```python
from build123d import *

# Parameters (mm, degrees)
F2_R          = 1.5875
F3_DEPTH      = 19.3685
F3_DEPTH_BACK = 19.3685
F6_W          = 76.2
F6_H          = 6.35
F7_DEPTH      = 5.438244135


with BuildPart() as f1:
    # F0 (on Front) → F1 (revolve)
    with BuildSketch(Plane.XZ):
        Polygon((72.6948, 19.3675), (0, 19.3675), (0, 14.2875), (85.3948, 14.2875), (85.3948, 18.0326762121), align=None)
    revolve(axis=Axis((42.6974, 0, 0), (1, 0, 0)))

    # F2 (on Front) → F3 (cut, two sides)
    with BuildSketch(Plane.XZ) as f3_sk:
        with Locations((82.8548, 0)):
            Circle(F2_R)
    extrude(amount=-F3_DEPTH, mode=Mode.SUBTRACT)
    extrude(f3_sk.sketch, amount=F3_DEPTH_BACK, mode=Mode.SUBTRACT)

    # F6 (on plane+point) → F7 (cut, through all)
    with BuildSketch(Plane.XY.offset(-19.3675)):
        with Locations((38.1, 0)):
            Rectangle(F6_W, F6_H)
        with BuildLine():
            ThreePointArc((76.2, -3.175), (79.375, 0), (76.2, 3.175))
            Line((76.2, 3.175), (76.2, -3.175))
        make_face()
    extrude(amount=F7_DEPTH, mode=Mode.SUBTRACT)


solid = f1.part
```
Geometry: final body of the model. Coordinates: model frame, mm. A direction names the side the tool comes from. Coordinates: 2 decimals unless noted, no trailing zeros. Loops run counter-clockwise (first coordinate to the right, second up) from the corner with the lowest first, then second, coordinate; pieces in that order, holes last. Notation, with made-up numbers: (-11, -25) -> (15, -25) arc R19 ccw to (15, -5) -> close; hole circle Ø10 at (35, -28). An arc over 180 degrees is marked (long way). Use a Markdown table: item, result. Add a question column.
(1) Section query A-A, the plane z = 0. Return loops of the section in (x, y).
(2) Section query B-B, the plane x = 69. Return loops of the section in (y, z) (1 decimal).
(3) Pin query (flat end, axial travel): pin 1 Ø4 at (x, z) = (28.5, -17) entering from -Y; pin 2 Ø2.5 at (x, z) = (53, -16) entering from +Y; pin 3 Ø4 at (x, y) = (59, -11.5) entering from -Z. Return the tip coordinate at first contact, or that it passes through.
(4) Access query for faces 1 (the conical face through (80.367, -5.575, 17.704)), 2 (the cylindrical face through (79.374, -0.07, -16.365)). Directions: +Z, -Z, +X, -X, +Y, -Y. A direction counts if a zero-diameter tool reaches every point of the face in a straight line with its end or side. Return the directions, or none.
(5) Line query: line 1 along Y through (x, z) = (19.5, 0); line 2 along X through (y, z) = (17.3, 0); line 3 along Z through (x, y) = (11, -6). Output: solid intervals per line, ascending.
(6) Mould query, pull axis Z, two halves, no side actions, for faces 3 (the flat face through (0, -3, 14.3)), 4 (the cylindrical face through (81.27, -16.3, 0.07)), 5 (the cylindrical face through (35.84, 0.81, 19.35)). Classes: pulls with the +Z half, pulls with the -Z half, needs draft (parallel to the pull), parting line crosses it, or undercut.
Answer:
| question | item | result |
|---|---|---|
| 1 | outline | (0, -19.37) -> (72.69, -19.37) -> (81.27, -18.47) -> (81.27, -14.29) -> (0, -14.29) -> close; (0, 14.29) -> (81.27, 14.29) -> (81.27, 18.47) -> (72.69, 19.37) -> (0, 19.37) -> close; (84.44, -18.13) -> (85.39, -18.03) -> (85.39, -14.29) -> (84.44, -14.29) -> close; (84.44, 14.29) -> (85.39, 14.29) -> (85.39, 18.03) -> (84.44, 18.13) -> close |
| 2 | outline | (-3.2, -19.1) -> (-3.2, -13.9) arc R14.3 cw (long way) to (3.2, -13.9) -> (3.2, -19.1) arc R19.4 ccw (long way) to start |
| 3 | pin 1 | stops at y = -12.25 |
| 3 | pin 2 | stops at y = 12.55 |
| 3 | pin 3 | stops at z = -16.88 |
| 4 | face 1 | +X |
| 4 | face 2 | -Z, -X |
| 5 | line 1 | y = -19.37 to -14.29, 14.29 to 19.37 |
| 5 | line 2 | x = 0 to 81.27, 84.44 to 85.39 |
| 5 | line 3 | z = -18.41 to -12.97, 12.97 to 18.41 |
| 6 | face 3 | needs draft |
| 6 | face 4 | undercut |
| 6 | face 5 | parting line crosses it |
